Could you check a few things on this model? Use its own coordinates, in mm. Give positions to 0.01 mm unless a question says otherwise; leave off trailing zeros. Order: outer loops, then holes, each group sorted by start corner. A loop starts at its lowest first (then second) coordinate and runs counter-clockwise, first axis right, second up. Notation, with made-up numbers: M 72,-11.75 L 102,-11.75 A34 ccw 102,20.25 Z; hole C 6.5,68 d10. An arc over 180 degrees is marked long. Use a Markdown table: item, result. Add a question column.
Item 1: I'm going to push flat-ended pins straight in: pin 1 Ø3 at (x, y) = (-28.14, 11.16) entering from -Z; pin 2 Ø2 at (y, z) = (80.5, 2.5) entering from -X; pin 3 Ø3 at (y, z) = (-37, 4) entering from +X; pin 4 Ø4.5 at (x, y) = (-77.5, 86.01) entering from +Z. Where does each tip first touch, or does it pass through?
Item 2: Suppose I cut it at B-B on z = 2.5. Count the separate pieces of the cut face and the enclosed holes in it, plus the area to 3 significant figures.
Item 3: Suppose I cut it at C-C on y = -24. Write out the boundary of the cut face in (x, z), plus the area to 4 significant figures.
Item 4: If I drill on L1, parallel to X at y = 87, z = 1.5; L2, parallel to Y at x = 0, z = 1.5; L3, parallel to X at y = 31, z = 6, over which ranges is the centre line in solid material (lowest first)? Write a range as from..to.
Item 5: Suppose I cut it at D-D on x = 0. Write out the boundary of the cut face in (y, z).
Item 6: Suppose I cut it at A-A on x = -77.5. Write out the boundary of the cut face in (y, z).
from build123d import *

# Parameters (mm, degrees)
BOSS_EXTRU_1_DEPTH      = 6.35
ENL_V_MAT_EXTRU_2_DEPTH = 144.087124508
ESQUISSE5_R             = 1.75
ENL_V_MAT_EXTRU_3_DEPTH = 100.149703595
BOSS_EXTRU_2_DEPTH      = 6.35
ESQUISSE11_R            = 2
ENL_V_MAT_EXTRU_4_DEPTH = 138.111345481


with BuildPart() as part:
    # Esquisse2 → Boss.-Extru.1 (new body)
    with BuildSketch(Plane.XY):
        Polygon((-71.473076574, 0), (71.473076574, 0), (0, 123.795), align=None)
    extrude(amount=BOSS_EXTRU_1_DEPTH)

    # Esquisse4 → Enlèv. mat.-Extru.2 (cut, through all)
    with BuildSketch(Plane.XY.offset(6.35)):
        Polygon((-71.473076574, 0), (-49.473076574, 38.105117767), (-27.473076574, 0), align=None)
        Polygon((71.473076574, 0), (27.473076574, 0), (49.473076574, 38.105117767), align=None)
        Polygon((0, 123.795), (-22, 85.689882233), (22, 85.689882233), align=None)
    extrude(amount=-ENL_V_MAT_EXTRU_2_DEPTH, mode=Mode.SUBTRACT)

    # Esquisse5 → Enlèv. mat.-Extru.3 (cut, through all)
    with BuildSketch(Plane.XY.offset(6.35)):
        with Locations((-40.142949555, 31.944863729)):
            Circle(ESQUISSE5_R)
        with Locations((-28.142949555, 11.160254038)):
            Circle(ESQUISSE5_R)
        with Locations((28.142949555, 11.160254038)):
            Circle(ESQUISSE5_R)
        with Locations((40.142949555, 31.944863729)):
            Circle(ESQUISSE5_R)
        with Locations((-12, 80.689882233)):
            Circle(ESQUISSE5_R)
        with Locations((12, 80.689882233)):
            Circle(ESQUISSE5_R)
    extrude(amount=-ENL_V_MAT_EXTRU_3_DEPTH, mode=Mode.SUBTRACT)

    # Esquisse10 → Boss.-Extru.2 (add)
    with BuildSketch(Plane(origin=(0, 0, 0), x_dir=(-1, 0, 0), z_dir=(0, 0, -1))):
        with BuildLine():
            Line((49.473076574, 38.105117767), (61.946156702, 59.709120804))
            Line((61.946156702, 59.709120804), (85.000000578, 73.019265173))
            ThreePointArc((85.000000578, 73.019265173), (90.4903807, 93.50964648), (69.999999393, 99.000026602))
            Line((69.999999393, 99.000026602), (46.946155518, 85.689882233))
            Line((46.946155518, 85.689882233), (22, 85.689882233))
            Line((22, 85.689882233), (49.473076574, 38.105117767))
        make_face()
        with BuildLine():
            Line((-22, 85.689882233), (-46.946155518, 85.689882233))
            Line((-46.946155518, 85.689882233), (-69.999999408, 99.000026577))
            ThreePointArc((-69.999999408, 99.000026577), (-90.490381043, 93.509645854), (-84.999999408, 73.019264463))
            Line((-84.999999408, 73.019264463), (-61.946154333, 59.709122172))
            Line((-61.946154333, 59.709122172), (-49.473076574, 38.105117767))
            Line((-49.473076574, 38.105117767), (-22, 85.689882233))
        make_face()
        with BuildLine():
            Line((-27.473076574, 0), (-15, -21.604005089))
            Line((-15, -21.604005089), (-15, -48.224291724))
            ThreePointArc((-15, -48.224291724), (0, -63.224291724), (15, -48.224291724))
            Line((15, -48.224291724), (15, -21.604005089))
            Line((15, -21.604005089), (27.473076574, 0))
            Line((27.473076574, 0), (-27.473076574, 0))
        make_face()
    extrude(amount=-BOSS_EXTRU_2_DEPTH)

    # Esquisse11 → Enlèv. mat.-Extru.4 (cut, through all)
    with BuildSketch(Plane.XY.offset(6.35)):
        with Locations((-77.5, 86.009645862)):
            Circle(ESQUISSE11_R)
        with Locations((77.5, 86.009645862)):
            Circle(ESQUISSE11_R)
        with Locations((0, -48.224291724)):
            Circle(ESQUISSE11_R)
    extrude(amount=-ENL_V_MAT_EXTRU_4_DEPTH, mode=Mode.SUBTRACT)


solid = part.part
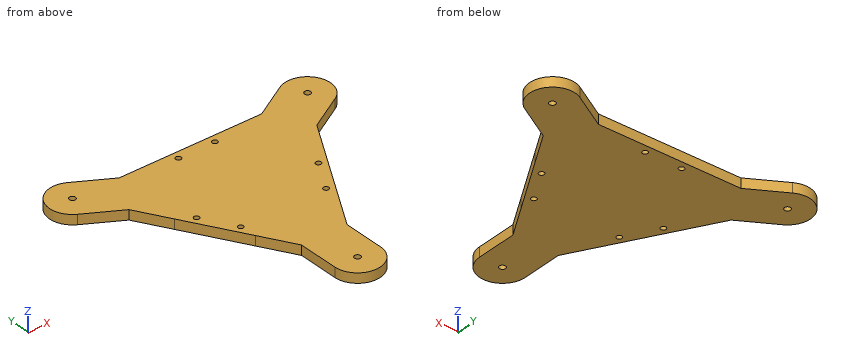
Findings below:
| question | item | result |
|---|---|---|
| 1 | pin 1 | passes through |
| 1 | pin 2 | stops at x = -91.81 |
| 1 | pin 3 | stops at x = 15 |
| 1 | pin 4 | stops at z = 6.35 |
| 2 | separate pieces | 1 |
| 2 | enclosed holes | 9 |
| 2 | area | 12,400 mm^2 |
| 3 | outline | M -15,0 L 15,0 L 15,6.35 L -15,6.35 Z |
| 3 | area | 190.5 mm^2 |
| 4 | L1 | x = -92.47..-79.24, -75.76..-49.22, 49.22..75.76, 79.24..92.47 |
| 4 | L2 | y = -63.22..-50.22, -46.22..85.69 |
| 4 | L3 | x = -45.37..-41.62, -38.67..38.67, 41.62..45.37 |
| 5 | outline | M -63.22,0 L -50.22,0 L -50.22,6.35 L -63.22,6.35 Z; M -46.22,0 L 85.69,0 L 85.69,6.35 L -46.22,6.35 Z |
| 6 | outline | M 68.69,0 L 84.01,0 L 84.01,6.35 L 68.69,6.35 Z; M 88.01,0 L 101.01,0 L 101.01,6.35 L 88.01,6.35 Z |
